Autodesk Inventor part; units mm, degrees
ref_plane "YZ Plane" through (0, 0, 0) normal (1, 0, 0) x (0, 1, 0)
ref_plane "XZ Plane" through (0, 0, 0) normal (0, 1, 0) x (-1, 0, 0)
ref_plane "XY Plane" through (0, 0, 0) normal (0, 0, 1) x (1, 0, 0)
sketch "Sketch1" plane through (0, 0, 0) normal (0, 1, 0) x (-1, 0, 0)
  circle A0 centre (0, 0) radius 17.4625
  line L0 (0, 0) -> (17.4625, 0) construction
  dimension "d0" = 34.925
extrude "Extrusion1" add sketch "Sketch1" along normal blind 3.175
sketch "Sketch2" plane through (0, 3.175, 0) normal (0, 1, 0) x (1, 0, 0)
  circle A0 centre (0, 0) radius 2
  line L0 (0, 0) -> (-14.2875, 0) construction
  arc A1 (-12.8229, 3.4359) -> (-12.8229, -3.4359) centre (-9.525, 0) ccw
  circle A2 centre (0, 0) radius 7.5 construction
  circle A3 centre (-7.5, 0) radius 1.5
  circle A4 centre (3.75, -6.4952) radius 1.5
  circle A5 centre (3.75, 6.4952) radius 1.5
  dimension "d10" = 15
  dimension "d9" = 4
  dimension "d11" = 3
  dimension "d14" = 360
extrude "Extrusion2" cut sketch "Sketch2" against normal through all
chamfer "Chamfer1" distance 3.175 angle 45 3 edges at (-9, 3.175, 0) (2.25, 3.175, -6.4952) (2.25, 3.175, 6.4952)
chamfer "Chamfer2" distance 1.5875 angle 45 1 edges at (17.4625, 3.175, 0)
properties part number "Hub Cap" material "Nylon 6/6"
Can you work these out from the model? Positions are in its coordinate system, mm. Give positions to 0.01 mm unless a question says otherwise; leave off trailing zeros. Return JSON: item names as keys, results as strings.
1. I want a section at A-A on z = 0. Give the number of separate pieces and of enclosed holes in the cut face, and give its area (3 significant figures).
Output values:
{"separate pieces": "3", "enclosed holes": "0", "area": "76.1 mm²"}
2. I'm going to push flat-ended pins straight in: pin 1 Ø1.5 at (y, z) = (2, 9.5) entering from -X; pin 2 Ø6 at (x, z) = (5, 7) entering from +Y. Where does each tip first touch, or does it pass through?
Output values:
{"pin 1": "stops at x = -15.04", "pin 2": "stops at y = 2.85"}
3. If I drill on line 1 (Z direction, x = 5.5, y = 0.75); line 2 (X direction, y = 2.9, z = -1.5); line 3 (Z direction, x = 5, y = 1.85), over which ranges is the centre line in solid material (lowest first)?
Output values:
{"line 1": "z = -16.57 to -7.91, -5.08 to 5.08, 7.91 to 16.57", "line 2": "x = -16.08 to -11.64, -3.36 to -1.32, 1.32 to 16.08", "line 3": "z = -16.46 to -9.6, -3.39 to 3.39, 9.6 to 16.46"}
4. We'd pull the mould along Z, two halves only. Please class faces 1 (the face through (0, 2, 2)), 2 (the face through (0, 3.175, -3)), 3 (the face through (13.858, 0.783, 10.626)): +Z half, -Z half, draft (parallel to the pull), parting line (faces both ways), or undercut.
Output values:
{"face 1": "undercut", "face 2": "draft", "face 3": "parting line"}
